```python
from build123d import *

# Parameters (mm, degrees)
F1_DEPTH = 63.5
F2_DEPTH = 25.4
F3_DEPTH = 7.9375
F0_W     = 15.7855516109
F0_H     = 19.05
F5_R     = 6.35


with BuildPart() as f1:
    # F0 (on Front) → F1 (new body, symmetric)
    with BuildSketch(Plane.XZ):
        Polygon((-41.275, 9.525), (-41.275, -9.525), (41.275, -9.525), (41.275, 9.525), (22.225, 9.525), align=None)
    extrude(amount=F1_DEPTH, both=True)

    # F0 (on Front) → F2 (join, symmetric)
    with BuildSketch(Plane.XZ):
        with BuildLine():
            Line((22.225, 9.525), (41.275, 9.525))
            Line((41.275, 9.525), (41.275, 27.0002))
            ThreePointArc((41.275, 27.0002), (45.9246798487, 38.2255201513), (57.15, 42.8752))
            Line((57.15, 42.8752), (60.325, 42.8752))
            Line((60.325, 42.8752), (60.325, 61.9252))
            Line((60.325, 61.9252), (57.15, 61.9252))
            add(Edge.make_bspline(
                [(56.0507958514, 61.9078979367), (56.4168804985, 61.9147360597), (56.7832864431, 61.9205050971), (57.15, 61.9252)],
                knots=[110.7182330401, 110.7182330401, 110.7182330401, 110.7182330401, 111.5045361635, 111.5045361635, 111.5045361635, 111.5045361635], degree=3))
            ThreePointArc((56.0507958514, 61.9078979367), (32.0686789633, 51.3041700472), (22.225, 27.0002))
            Line((22.225, 27.0002), (22.225, 9.525))
        make_face()
    extrude(amount=F2_DEPTH, both=True)

    # F0 (on Front) → F3 (join, symmetric)
    with BuildSketch(Plane.XZ):
        with BuildLine():
            add(Edge.make_bspline(
                [(-41.275, 9.525), (-40.6745437573, 38.785344003), (4.5029333836, 60.945031492), (56.0507958514, 61.9078979367)],
                knots=[0, 0, 0, 0, 110.7182330401, 110.7182330401, 110.7182330401, 110.7182330401], degree=3))
            Line((-41.275, 9.525), (22.225, 9.525))
            Line((22.225, 9.525), (22.225, 27.0002))
            ThreePointArc((22.225, 27.0002), (32.0686789633, 51.3041700472), (56.0507958514, 61.9078979367))
        make_face()
    extrude(amount=F3_DEPTH, both=True)

    # F0 (on Front) → F4 (revolve)
    with BuildSketch(Plane.XZ):
        with Locations((68.2177758054, 52.4002)):
            Rectangle(F0_W, F0_H)
    revolve(axis=Axis((60.325, 0, 52.3875), (0, 0, 1)))

    # F5
    f5_edges = [f1.edges().sort_by_distance(p)[0] for p in [
        (41.275, -63.5, 0),
        (-41.275, -63.5, 0),
        (41.275, 63.5, 0),
        (-41.275, 63.5, 0),
    ]]
    fillet(f5_edges, radius=F5_R)


solid = f1.part
```
Geometry: final body of the model. Coordinates: model frame, mm. A direction names the side the tool comes from. Give positions to 0.01 mm unless a question says otherwise; leave off trailing zeros. Loops run counter-clockwise (first coordinate to the right, second up) from the corner with the lowest first, then second, coordinate; pieces in that order, holes last. Notation, with made-up numbers: (-38.75, 59.5) - (-34.75, 59.5) arc R31 ccw to (-34.75, 83.5) - close; hole circle Ø11 at (50.5, 89.5). An arc over 180 degrees is marked (long way). Answer as CSV lines item,"result". Start each with the question number.
(1) Pin query (flat end, axial travel): P1, Ø2, axis at x = 54.5, y = -24, coming from the -Z side; P2, Ø14, axis at y = -20, z = 19.5, coming from the -X side (3 decimals); P3, Ø5, axis at y = -9.5, z = 27, coming from the -X side. Return the tip coordinate at first contact, or that it passes through.
(2) Ray query, line 1 along Z through (x, y) = (-11, 36.5) (3 decimals); line 2 along Y through (x, z) = (10, 42); line 3 along X through (y, z) = (-31, 8) (3 decimals). Return the intervals inside material, ascending. Write a range as [from, to].
(3) Section query C-C (y = -42). Output: boundary loops of the cut face in (x, z) (3 decimals), and give its area (3 significant figures).
(4) Section query B-B (y = 13). Output: boundary loops of the cut face in (x, z) (3 decimals).
(5) Reachability of faces 1 (the face through (32.33, 16.55, 51.57)), 2 (the face through (65, 0, 42.875)), 3 (the face through (22.225, -17, 18)) from +Z, -Z, +X, -X, +Y, -Y: full face, straight path, thin tool, end or side. Return the list, or none.
(6) Section query A-A (x = 52.5). Output: boundary loops of the cut face in (y, z), and give its area (3 significant figures).
Worked answers:
1,P1,"stops at z = 42.45"
1,P2,"stops at x = 22.225"
1,P3,"stops at x = -36.54"
2,line 1,"z = [-9.525, 9.525]"
2,line 2,"y = [-7.94, 7.94]"
2,line 3,"x = [-41.275, 41.275]"
3,outline,"(-41.275, -9.525) - (41.275, -9.525) - (41.275, 9.525) - (-41.275, 9.525) - close"
3,area,"1,570 mm^2"
4,outline,"(-41.275, -9.525) - (41.275, -9.525) - (41.275, 27) arc R15.875 cw to (57.15, 42.875) - (69.28, 42.875) - (69.28, 61.925) - (51.37, 61.925) - (51.37, 61.444) arc R34.925 ccw to (22.225, 27) - (22.225, 9.525) - (-41.275, 9.525) - close"
5,face 1,"+Z, -X, +Y"
5,face 2,"-Z, +X, +Y, -Y"
5,face 3,"+Z, -X, -Y"
6,outline,"(-25.4, 42.18) - (25.4, 42.18) - (25.4, 61.61) - (13.71, 61.61) - (13.71, 61.93) - (-13.71, 61.93) - (-13.71, 61.61) - (-25.4, 61.61) - close"
6,area,"996 mm^2"
